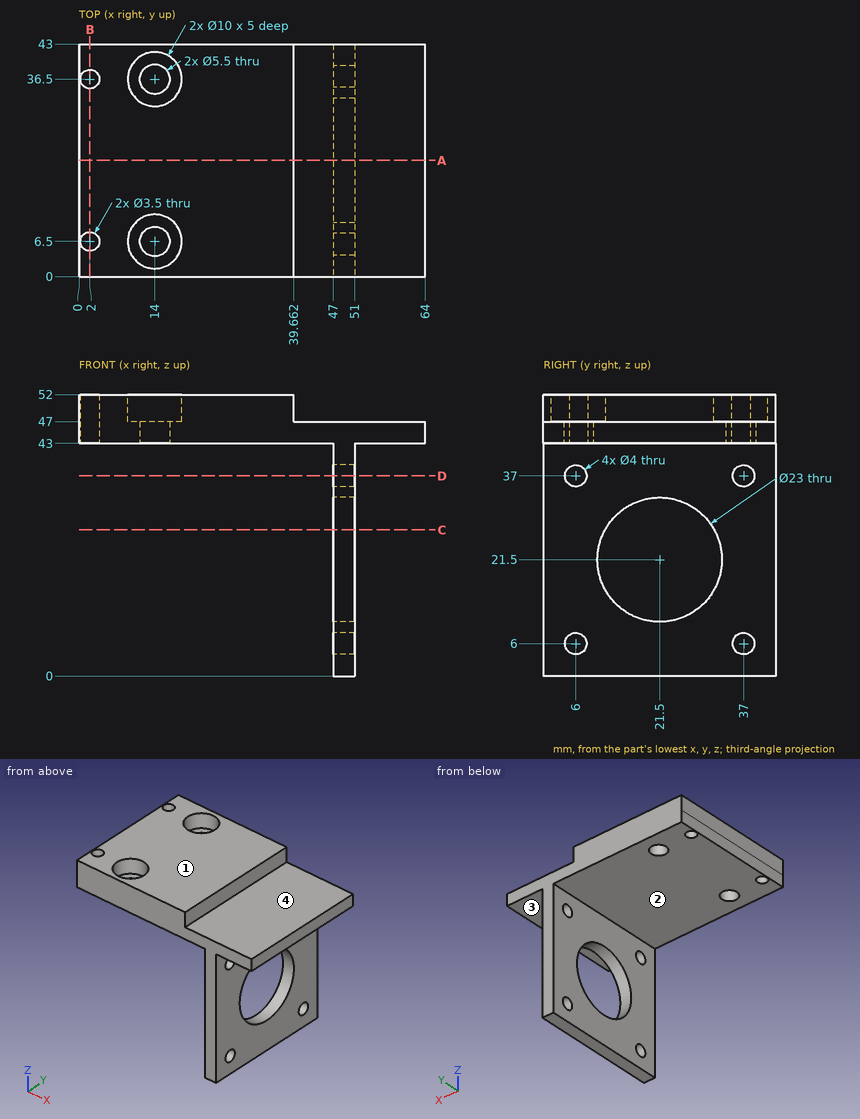
Could you check a few things on this drawing? It's one solid part, dimensions in mm from its lowest x, y, z. A direction names the side the tool comes from. Coordinates: 2 decimals unless noted, no trailing zeros. Order: outer loops, then holes, each group sorted by start corner. A loop starts at its lowest first (then second) coordinate and runs counter-clockwise, first axis right, second up. Notation, with made-up numbers: M -24,11.5 L 5,11.5 A23 ccw 5,28.5 Z; hole C 47,37.5 d7. An arc over 180 degrees is marked long. Use a Markdown table: item, result. Add a question column.
Q1. I want a section at C-C on z = 27. List the corners of the cut face in (x, y) for me.
Q2. I'm going to push flat-ended pins straight in: pin 1 (10.5 mm diameter, centred on x = 58, y = 19, fed in from -Z); pin 2 (7 mm diameter, centred on x = 14, y = 6.5, fed in from +Z); pin 3 (21.5 mm diameter, centred on y = 16.5, z = 11, fed in from -X). Where does each tip first touch, or does it pass through?
Q3. If I drill on L1, parallel to Z at x = 48.25, y = 37; L2, parallel to Y at x = 14, z = 50.15; L3, parallel to Y at x = 2, z = 47, over which ranges is the centre line in solid material (lowest first)?
Q4. I want a section at D-D on z = 37. List the corners of the cut face in (x, y) for me.
Q5. I want a section at A-A on y = 21.5. List the corners of the cut face in (x, z) for me.
Q6. Which directions (+Z, -Z, +X, -X, +Y, -Y) give clear straight access to the entire face, cutting with the end or side of a thin tool? Please do the marked faces 1, 2, 3 and 4.
Q7. I want a section at B-B on x = 2. List the corners of the cut face in (y, z) for me.
Checked values:
| question | item | result |
|---|---|---|
| 1 | outline | M 47,0 L 51,0 L 51,11.4 L 47,11.4 Z; M 47,31.6 L 51,31.6 L 51,43 L 47,43 Z |
| 2 | pin 1 | z = 43 |
| 2 | pin 2 | z = 47 |
| 2 | pin 3 | x = 47 |
| 3 | L1 | 0 to 4, 8 to 35, 39 to 47 |
| 3 | L2 | 0 to 1.5, 11.5 to 31.5, 41.5 to 43 |
| 3 | L3 | 0 to 4.75, 8.25 to 34.75, 38.25 to 43 |
| 4 | outline | M 47,0 L 51,0 L 51,4 L 47,4 Z; M 47,8 L 51,8 L 51,35 L 47,35 Z; M 47,39 L 51,39 L 51,43 L 47,43 Z |
| 5 | outline | M 0,43 L 47,43 L 47,33 L 51,33 L 51,43 L 64,43 L 64,47 L 39.66,47 L 39.66,52 L 0,52 Z; M 47,0 L 51,0 L 51,10 L 47,10 Z |
| 6 | face 1 | +Z, +X, -X, +Y, -Y |
| 6 | face 2 | -Z, -X, +Y, -Y |
| 6 | face 3 | -Z, +X, +Y, -Y |
| 6 | face 4 | +Z, +X, +Y, -Y |
| 7 | outline | M 0,43 L 4.75,43 L 4.75,52 L 0,52 Z; M 8.25,43 L 34.75,43 L 34.75,52 L 8.25,52 Z; M 38.25,43 L 43,43 L 43,52 L 38.25,52 Z |
